The listing builds one solid part. Answer for the finished solid, in the listing's coordinates (mm). Face numbers are marked on the shaded views. A direction names the side the tool comes from. Round coordinates to 2 decimals unless told otherwise and drop trailing zeros. Write each loop counter-clockwise with the first axis right and the second up, starting at its lowest first coordinate (ties: lowest second). Pieces come first, ordered by that corner, then holes. Notation, with made-up numbers: (86, 35.5) - (106, 35.5) arc R24 ccw to (106, 53.5) - close; hole circle Ø2 at (-38, -15.75). An arc over 180 degrees is marked (long way). Use a Markdown table: item, result. Add a question column.
1) A cutting plane is placed at A-A (y = 25). Give the vertices of the cut face in (x, z).
2) A cutting plane is placed at B-B (x = 2.3). Give the vertices of the cut face in (y, z) (3 decimals).
3) A cutting plane is placed at D-D (z = 30.5). Give the vertices of the cut face in (x, y) (3 decimals).
4) A cutting plane is placed at C-C (z = 0). Give the vertices of the cut face in (x, y).
5) Each of these flat-tipped pins is pushed along its axis until it touches: P1, Ø1.5, axis at x = 2, z = 13, coming from the +Y side (3 decimals); P2, Ø0.6, axis at x = 3.5, z = 14.5, coming from the -Y side (3 decimals); P3, Ø8, axis at y = -25, z = 0, coming from the -X side; P4, Ø5, axis at y = 0, z = 0, coming from the -X side. Where does it stop, or does it pass through?
6) A tool of negligible diameter and unlimited length cuts with its end or side. For the marked faces 4, 5 and 6, from which of +Z, -Z, +X, -X, +Y, -Y can it reach the whole face along a straight path? Write none if from no direction.
7) Determine the mould class of the marked faces 1, 2 and 3 for opening direction X: +X half, -X half, draft (parallel to the pull), parting line (faces both ways), or undercut.
8) Find the intervals of material crossed by probe 1 along Y at (x, z) = (4.05, 15.5) (3 decimals); probe 2 along Z at (x, y) = (1.7, 25); probe 3 along Y at (x, z) = (1.95, 19.5) (3 decimals), in increasing order. Write a range as from..to.
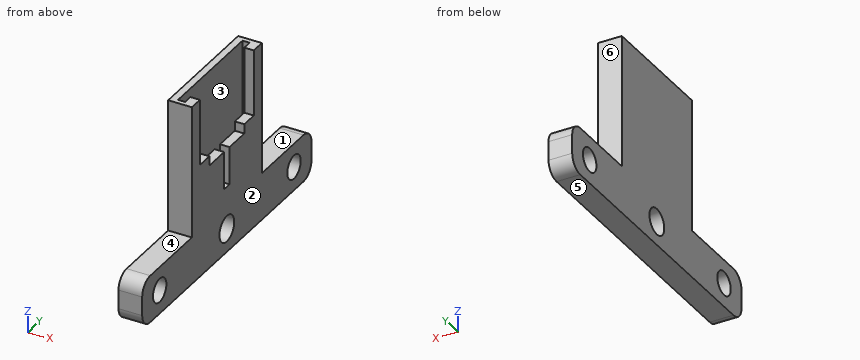
```python
from build123d import *

# Parameters (mm, degrees)
F0_R     = 2.5
F1_DEPTH = 5
F2_D     = 5.5
F2_DEPTH = 7
F2_TIP   = 1.6523667023
F4_DEPTH = 5
F6_DEPTH = 3.5
F7_W     = 1.5
F7_H     = 1.975
F8_DEPTH = 24


with BuildPart() as f1:
    # F0 (on Right) → F1 (new body)
    with BuildSketch(Plane.YZ):
        with BuildLine():
            Line((-28.5, -5), (28.5, -5))
            ThreePointArc((28.5, -5), (30.6213203436, -4.1213203436), (31.5, -2))
            Line((31.5, -2), (31.5, 2))
            ThreePointArc((31.5, 2), (30.6213203436, 4.1213203436), (28.5, 5))
            Line((28.5, 5), (-28.5, 5))
            ThreePointArc((-28.5, 5), (-30.6213203436, 4.1213203436), (-31.5, 2))
            Line((-31.5, 2), (-31.5, -2))
            ThreePointArc((-31.5, -2), (-30.6213203436, -4.1213203436), (-28.5, -5))
        make_face()
        with Locations((-25, 0)):
            Circle(F0_R, mode=Mode.SUBTRACT)
        with Locations((25, 0)):
            Circle(F0_R, mode=Mode.SUBTRACT)
    extrude(amount=F1_DEPTH)

    # F2
    with Locations(Plane(origin=(0, 0, 0), x_dir=(0, 1, 0), z_dir=(-1, 0, 0))):
        with Locations((0, 0)):
            Hole(F2_D / 2, depth=F2_DEPTH)
            with Locations((0, 0, -(F2_DEPTH + F2_TIP / 2))):  # 118° drill point
                Cone(0, F2_D / 2, F2_TIP, mode=Mode.SUBTRACT)

    # F3 (on Right) → F4 (join, through all)
    with BuildSketch(Plane.YZ):
        Polygon((-13.025, 33), (-13.025, 5), (13.025, 5), (13.025, 33), (0, 33), align=None)
    extrude(amount=F4_DEPTH)

    # F5 (on face) → F6 (cut)
    with BuildSketch(Plane.YZ.offset(5)):
        Polygon((10.025, 33), (-10.025, 33), (-10.025, 19), (-6.5, 19), (-6.5, 17), (-1, 17), (-1, 9), (1, 9), (1, 17), (6.5, 17), (6.5, 19), (10.025, 19), align=None)
    extrude(amount=-F6_DEPTH, mode=Mode.SUBTRACT)

    # F7 (on face) → F8 (cut, through all)
    with BuildSketch(Plane.XY.offset(33)):
        Polygon((1.5, 10.025), (1.5, 0), (1.5, -10.025), (3, -10.025), (3, 0), (3, 10.025), align=None)
        with Locations((2.25, -11.0125)):
            Rectangle(F7_W, F7_H)
        with Locations((2.25, 11.0125)):
            Rectangle(F7_W, F7_H)
    extrude(amount=-F8_DEPTH, mode=Mode.SUBTRACT)


solid = f1.part
```
Entries:
| question | item | result |
|---|---|---|
| 1 | outline | (0, -5) - (5, -5) - (5, -2.5) - (0, -2.5) - close; (0, 2.5) - (5, 2.5) - (5, 5) - (0, 5) - close |
| 2 | outline | (-31.5, -2) arc R3 ccw to (-28.5, -5) - (28.5, -5) arc R3 ccw to (31.5, -2) - (31.5, 2) arc R3 ccw to (28.5, 5) - (13.025, 5) - (13.025, 33) - (12, 33) - (12, 9) - (-12, 9) - (-12, 33) - (-13.025, 33) - (-13.025, 5) - (-28.5, 5) arc R3 ccw to (-31.5, 2) - close; hole circle Ø5 at (-25, 0); hole circle Ø5.5 at (0, 0); hole circle Ø5 at (25, 0) |
| 3 | outline | (0, -13.025) - (5, -13.025) - (5, -10.025) - (3, -10.025) - (3, -12) - (1.5, -12) - (1.5, 12) - (3, 12) - (3, 10.025) - (5, 10.025) - (5, 13.025) - (0, 13.025) - close |
| 4 | outline | (0, -31.5) - (5, -31.5) - (5, -27.5) - (0, -27.5) - close; (0, -22.5) - (5, -22.5) - (5, -2.75) - (0, -2.75) - close; (0, 2.75) - (5, 2.75) - (5, 22.5) - (0, 22.5) - close; (0, 27.5) - (5, 27.5) - (5, 31.5) - (0, 31.5) - close |
| 5 | P1 | stops at y = 13.025 |
| 5 | P2 | stops at y = -13.025 |
| 5 | P3 | stops at x = 0 |
| 5 | P4 | passes through |
| 6 | face 4 | +Z, +X, -X, -Y |
| 6 | face 5 | -Z, +X, -X, +Y, -Y |
| 6 | face 6 | +Z, +X, -X, +Y |
| 7 | face 1 | draft |
| 7 | face 2 | +X half |
| 7 | face 3 | undercut |
| 8 | probe 1 | y = -13.025..-1, 1..13.025 |
| 8 | probe 2 | z = -5..-2.5, 2.5..5 |
| 8 | probe 3 | y = -13.025..-12, 12..13.025 |
